Check sheet for the modelled part. Datum: model origin and axes. Units: mm. Face numbers are marked on the shaded views. A direction names the side the tool comes from. Give positions to 0.01 mm unless a question says otherwise; leave off trailing zeros. Write each loop counter-clockwise with the first axis right and the second up, starting at its lowest first coordinate (ties: lowest second). Pieces come first, ordered by that corner, then holes.
from build123d import *

# Parameters (mm, degrees)
F_2_0_2_DIAMETER_HOLE1_D           = 2
F_2_0_2_DIAMETER_HOLE1_CSINK_D     = 2.05
F_2_0_2_DIAMETER_HOLE1_CSINK_ANGLE = 90


with BuildPart() as part:
    # Sketch1 → Revolve1 (revolve)
    with BuildSketch(Plane.XY):
        Polygon((9.549685022, 1.278125845), (9.549685022, 2.528125845), (-2.450314978, 2.528125845), (-3.950314978, 2.528125845), (-3.950314978, 1.028125845), (-11.950314978, 1.028125845), (-11.950314978, -0.471874155), (-2.450314978, -0.471874155), (-2.450314978, 1.028125845), (1.549685022, 1.028125845), (1.549685022, 1.278125845), align=None)
    revolve(axis=Axis((0, -1.971874155, 0), (-1, 0, 0)))

    # Ø2.0 (2) Diameter Hole1 (through all)
    with Locations(Plane(origin=(4.068165659, -1.965730097, 4.499995806), x_dir=(0, 0.999999068, -0.001365346), z_dir=(0, 0.001365346, 0.999999068))):
        with Locations((0, 0)):
            CounterSinkHole(F_2_0_2_DIAMETER_HOLE1_D / 2, F_2_0_2_DIAMETER_HOLE1_CSINK_D / 2, counter_sink_angle=F_2_0_2_DIAMETER_HOLE1_CSINK_ANGLE)


solid = part.part
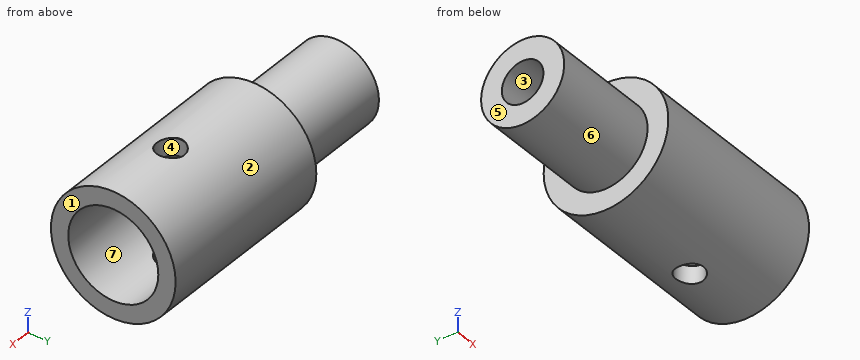
1) Draft check along Y on the marked faces 1, 2, 3 and 4. Enter one of: +Y half, -Y half, draft (parallel to the pull), parting line (faces both ways), or undercut.
2) Sectioned sample at C-C on x = -9.75. Record the boundary of the cut face in (y, z).
3) Sectioned sample at D-D on y = -1.25. Give the number of separate pieces and of enclosed holes in the cut face, then the cut area to 3 significant figures.
4) Scan lines: L1, parallel to Y at x = 0.5, z = 0; L2, parallel to Y at x = 3.5, z = 0; L3, parallel to X at y = 0, z = -0.5. Record each from-to range of solid material in increasing order.
5) Sectioned sample at A-A on z = 0. Record the boundary of the cut face in (x, y), then the cut area to 3 significant figures.
6) Sectioned sample at B-B on z = -2.5. Record the boundary of the cut face in (x, y), then the cut area to 3 significant figures.
7) Access from +Z, -Z, +X, -X, +Y, -Y to the whole of each face (thin tool, end or side, straight path). Record for the marked faces 5, 6 and 7.
8) Gauge pin test, flat ends, axial feed: pin 1 (5 mm diameter, centred on x = 1, y = 0, fed in from +Z); pin 2 (5 mm diameter, centred on y = -1.97, z = 0, fed in from +X); pin 3 (5 mm diameter, centred on x = 6, z = -3.5, fed in from -Y); pin 4 (3 mm diameter, centred on y = -2.5, z = -1.5, fed in from +X). Record the tip position at first contact, or that the pin passes through.
Answers below:
1. face 1: draft
1. face 2: parting line
1. face 3: undercut
1. face 4: undercut
2. outline: circle Ø6 at (-1.97, 0); hole circle Ø3 at (-1.97, 0)
3. separate pieces: 4
3. enclosed holes: 0
3. area: 64.0 mm2
4. L1: y = -6.47 to -4.97, 1.03 to 2.53
4. L2: y = -6.47 to -5.22, 1.28 to 2.53
4. L3: x = -11.95 to -2.45
5. outline: (-11.95, -4.97) - (-3.95, -4.97) - (-3.95, -6.47) - (9.55, -6.47) - (9.55, -5.22) - (1.55, -5.22) - (1.55, -4.97) - (-2.45, -4.97) - (-2.45, -3.47) - (-11.95, -3.47) - close; (-11.95, -0.47) - (-2.45, -0.47) - (-2.45, 1.03) - (1.55, 1.03) - (1.55, 1.28) - (9.55, 1.28) - (9.55, 2.53) - (-3.95, 2.53) - (-3.95, 1.03) - (-11.95, 1.03) - close
5. area: 65.0 mm2
6. outline: (-11.95, -3.63) - (-3.95, -3.63) - (-3.95, -5.71) - (9.55, -5.71) - (9.55, -4.05) - (1.55, -4.05) - (1.55, -3.63) - (-2.45, -3.63) - (-2.45, -0.31) - (1.55, -0.31) - (1.55, 0.1) - (9.55, 0.1) - (9.55, 1.77) - (-3.95, 1.77) - (-3.95, -0.31) - (-11.95, -0.31) - close
6. area: 81.1 mm2
7. face 5: +Z, -Z, -X, +Y, -Y
7. face 6: -X
7. face 7: +X
8. pin 1: stops at z = 4.5
8. pin 2: stops at x = -2.45
8. pin 3: stops at y = -6.36
8. pin 4: stops at x = 1.55
